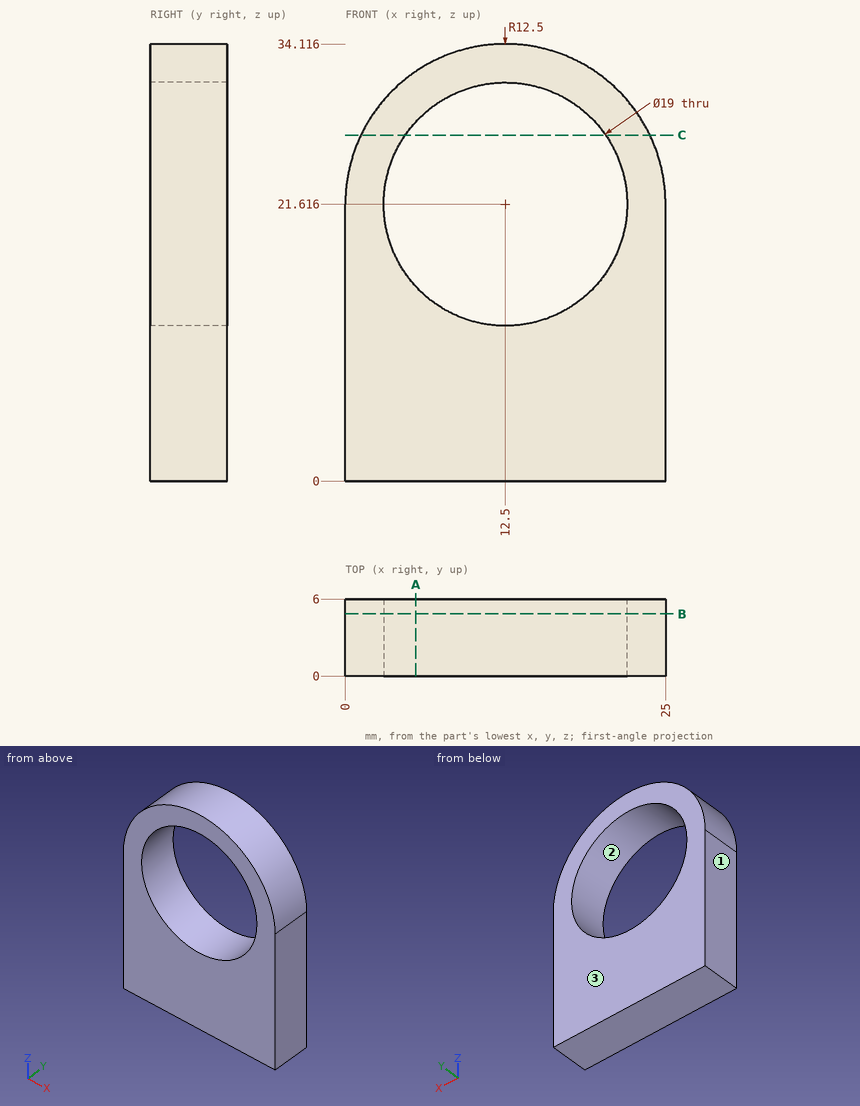
Source: three-view drawing plus pictorial views. Frame: mm from the lowest corner of the part. Coordinates: 2 decimals unless noted, no trailing zeros. Order: outer loops, then holes, each group sorted by start corner. A loop starts at its lowest first (then second) coordinate and runs counter-clockwise, first axis right, second up. Notation, with made-up numbers: (22, 66) -> (46, 66) arc R22 ccw to (46, 79) -> close; hole circle Ø4 at (32.25, 68). An arc over 180 degrees is marked (long way). Write item = value, one per line.
(1) Cut plane B-B on y = 4.85. Return loops of the section in (x, z).
Solved:
outline = (0, 0) -> (25, 0) -> (25, 21.62) arc R12.5 ccw to (0, 21.62) -> close; hole circle Ø19 at (12.5, 21.62)
(2) Pull-direction query (X, two-part tool) for the marked faces 1, 2 and 3; classes: pulls with the +X half, pulls with the -X half, needs draft (parallel to the pull), parting line crosses it, or undercut.
Solved:
face_1 = pulls with the -X half
face_2 = undercut
face_3 = needs draft
(3) Line query: line 1 (Z direction, x = 12.5, y = 1.95); line 2 (X direction, y = 2.95, z = 22); line 3 (X direction, y = 2.55, z = 23). Output: solid intervals per line, ascending.
Solved:
line_1 = 0 to 12.12, 31.12 to 34.12
line_2 = 0.01 to 3.01, 21.99 to 24.99
line_3 = 0.08 to 3.1, 21.9 to 24.92
(4) Cut plane C-C on z = 27. Return loops of the section in (x, y).
Solved:
outline = (1.22, 0) -> (4.67, 0) -> (4.67, 6) -> (1.22, 6) -> close; (20.33, 0) -> (23.78, 0) -> (23.78, 6) -> (20.33, 6) -> close
(5) Cut plane A-A on x = 5.5. Return loops of the section in (y, z).
Solved:
outline = (0, 0) -> (6, 0) -> (6, 15.19) -> (0, 15.19) -> close; (0, 28.04) -> (6, 28.04) -> (6, 31.97) -> (0, 31.97) -> close
(6) Pin query (flat end, axial travel): pin 1 Ø1 at (y, z) = (2, 28.5) entering from -X; pin 2 Ø3 at (y, z) = (4, 25.5) entering from -X. Return the tip coordinate at first contact, or that it passes through.
Solved:
pin_1 = 1.75
pin_2 = 0.23
